CAD build for the part. Positions are in the model's coordinates, mm. Coordinates: 2 decimals unless noted, no trailing zeros. Order: outer loops, then holes, each group sorted by start corner. A loop starts at its lowest first (then second) coordinate and runs counter-clockwise, first axis right, second up. Notation, with made-up numbers: M 41,77.5 L 51,77.5 A26 cw 51,114.5 Z; hole C 12.25,87 d10. An arc over 180 degrees is marked long. Write item = value, one per line.
from build123d import *


with BuildPart() as part:
    # Süpür1: sweep along a path in Çizim2
    with BuildLine(Plane(origin=(0, 0, 0), x_dir=(0, 0, -1), z_dir=(1, 0, 0))) as s_p_r1_path:
        Line((0, 0), (20, 0))
        ThreePointArc((20, 0), (23.535533906, -1.464466094), (25, -5))
        Line((25, -5), (25, -65))
    # Çizim1 → Süpür1 (sweep)
    with BuildSketch(Plane.XY):
        Polygon((1.732050808, 0), (0.866025404, 1.5), (-0.866025404, 1.5), (-1.732050808, 0), (-0.866025404, -1.5), (0.866025404, -1.5), align=None)
    sweep(path=s_p_r1_path.line)


solid = part.part
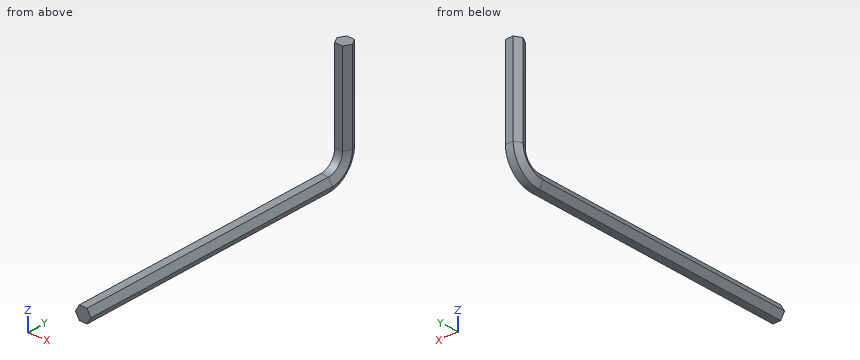
(1) Wall check: line 1 (Y direction, x = 0.15, z = -12.75); line 2 (Z direction, x = 0.2, y = -15.5); line 3 (Z direction, x = -1.45, y = -58.5). Give the ranges that are in metal, low to high. Write a range as from..to.
Evaluation:
line_1 = -1.5..1.5
line_2 = -26.5..-23.5
line_3 = -25.49..-24.51
(2) Slice it at A-A, the plane x = -0.05. Write the cut outline in (y, z).
Evaluation:
outline = M -65,-26.5 L -5,-26.5 A6.5 ccw 1.5,-20 L 1.5,0 L -1.5,0 L -1.5,-20 A3.5 cw -5,-23.5 L -65,-23.5 Z
(3) Slice it at C-C, the plane y = -58.5. Write the cut outline in (x, z).
Evaluation:
outline = M -1.73,-25 L -0.87,-26.5 L 0.87,-26.5 L 1.73,-25 L 0.87,-23.5 L -0.87,-23.5 Z
(4) Slice it at B-B, the plane z = -7.25. Write the cut outline in (x, y), then the cut area to 3 significant figures.
Evaluation:
outline = M -1.73,0 L -0.87,-1.5 L 0.87,-1.5 L 1.73,0 L 0.87,1.5 L -0.87,1.5 Z
area = 7.79 mm²
(5) Pin check, flat tips, straight feed: pin 1 Ø0.9 at (x, z) = (0.5, -7.5) entering from -Y; pin 2 Ø0.9 at (x, y) = (0, -35.5) entering from +Z; pin 3 Ø12 at (y, z) = (-5.5, -3) entering from +X. Stop position of each tip, or through.
Evaluation:
pin_1 = -1.5
pin_2 = -23.5
pin_3 = 1.73
